Could you check a few things on this model? Use its own coordinates, in mm. A direction names the side the tool comes from. Round coordinates to 2 decimals unless told otherwise and drop trailing zeros. Write each loop counter-clockwise with the first axis right and the second up, starting at its lowest first coordinate (ties: lowest second). Pieces come first, ordered by that corner, then holes. Notation, with made-up numbers: (-7.5, 73) -> (33.5, 73) arc R24 ccw to (33.5, 85) -> close; hole circle Ø1 at (-29, 50). An arc over 180 degrees is marked (long way). Answer in a Markdown table with one row per item. Add a question column.
```python
from build123d import *

# Parameters (mm, degrees)
PAD030_DEPTH         = 10
PAD041_DEPTH         = 1
SKETCH081_R          = 4
POCKET023_DEPTH      = 16.001
POCKET023_DEPTH_BACK = 16.001


with BuildPart() as part:
    # Sketch066 → Pad030 (new body, symmetric)
    with BuildSketch(Plane.YZ):
        with BuildLine():
            ThreePointArc((54.1777871717, -5.4865141741), (68, 0), (54.1777871717, 5.4865141741))
            ThreePointArc((47.2218073921, 2.3498355523), (51.010737248, 3.2286263383), (54.1777871717, 5.4865141741))
            Line((47.2218073921, 2.3498355523), (15.1843604449, 1.3183803873))
            Line((17.6038721988, 3.8988686334), (15.1843604449, 1.3183803873))
            Line((-12.580488246, 2.9270741413), (17.6038721988, 3.8988686334))
            Line((-10, 0.5075623873), (-12.580488246, 2.9270741413))
            Line((-10, 0.5075623873), (-18, 0.25))
            ThreePointArc((-13.7330991232, 6), (-16.8683496754, 3.8684055277), (-18, 0.25))
            Line((-13.7330991232, 6), (12.3912565298, 13))
            Line((12.3912565298, 13), (103.7477270849, 13))
            ThreePointArc((107.6207104311, 8), (110.7829880912, 14.4494897428), (103.7477270849, 13))
            Line((73.7477270849, 8), (107.6207104311, 8))
            ThreePointArc((73.7477270849, 8), (72.0744070318, 7.095445115), (71.9146968069, 5.2))
            ThreePointArc((71.9146968069, -5.2), (73, 0), (71.9146968069, 5.2))
            ThreePointArc((71.9146968069, -5.2), (72.0744070318, -7.095445115), (73.7477270849, -8))
            Line((73.7477270849, -8), (107.6207104311, -8))
            ThreePointArc((103.7477270849, -13), (110.7829880912, -14.4494897428), (107.6207104311, -8))
            Line((12.3912565298, -13), (103.7477270849, -13))
            Line((-13.7330991232, -6), (12.3912565298, -13))
            ThreePointArc((-18, -0.25), (-16.8683496754, -3.8684055277), (-13.7330991232, -6))
            Line((-18, -0.25), (-10, -0.5075623873))
            Line((-10, -0.5075623873), (-12.580488246, -2.9270741413))
            Line((-12.580488246, -2.9270741413), (17.6038721988, -3.8988686334))
            Line((17.6038721988, -3.8988686334), (15.1843604449, -1.3183803873))
            Line((15.1843604449, -1.3183803873), (47.2218073921, -2.3498355523))
            ThreePointArc((54.1777871717, -5.4865141741), (51.010737248, -3.2286263383), (47.2218073921, -2.3498355523))
        make_face()
    extrude(amount=PAD030_DEPTH, both=True)

    # Sketch082 (on Face28 of Pad030) → Pad041 (join)
    with BuildSketch(Plane.YZ.offset(10)):
        Polygon((-12.580488246, 2.9270741413), (-10, 0.5075623873), (15.1843604449, 1.3183803873), (17.6038721988, 3.8988686334), align=None)
        Polygon((-10, -0.5075623873), (15.1843604449, -1.3183803873), (17.6038721988, -3.8988686334), (-12.580488246, -2.9270741413), align=None)
    extrude(amount=-PAD041_DEPTH)

    # Sketch081 → Pocket023 (cut, two sides)
    with BuildSketch(Plane.XY) as pocket023_sk:
        Circle(SKETCH081_R)
    extrude(amount=-POCKET023_DEPTH, mode=Mode.SUBTRACT)
    extrude(pocket023_sk.sketch, amount=POCKET023_DEPTH_BACK, mode=Mode.SUBTRACT)


with BuildPart() as part_1:
    # Body021 placement: moved
    add(part.part.moved(Location((0, -2, 2.5))))


solid = part_1.part
```
(1) I need wall thicknesses on L1, parallel to Z at x = 4.25, y = 58; L2, parallel to Z at x = 5.5, y = -14; L3, parallel to Z at x = -6, y = 23. Which ranges of each line are inside material? Lowest first, please.
(2) Suppose I cut it at A-A, the plane y = 58. Please give me the cut outline in (x, z), then the cut area to 3 significant figures.
(3) If we mould it in two halves opening along Z, with no side actions, what happens to faces 6 (the face through (-0.521, 1.966, 8.58)), 7 (the face through (0.14, 70.06, -4.57)), 8 (the face through (-2.082, -5.756, 11.173)), 9 (the face through (-0.367, 14.411, 5.127))? For each: pulls with the +Z half, pulls with the -Z half, needs draft (parallel to the pull), parting line crosses it, or undercut.
(4) On a 3-axis mill with a long thin cutter (end or side, diameter ignored), from which of +Z, -Z, +X, -X, +Y, -Y can I reach the whole of each face in a straight line? I mean faces 1 (the face through (-2.082, -5.756, -6.173)), 2 (the face through (10, 29, 6)), 3 (the face through (0.14, 48.961, 5.706)), 4 (the face through (0, 88, 10.5)), 5 (the face through (9, 1, 0)). Say none if no direction works.
(5) Suppose I cut it at C-C, the plane x = -0.5. State how many separate pieces and enclosed holes the cut face has, then the cut area to 3 significant figures.
(6) Suppose I cut it at B-B, the plane y = -2. Please give me the cut outline in (x, z), then the cut area to 3 significant figures.
(7) For P1, Ø1, axis at x = 3, z = 12.5, coming from the -Y side; P2, Ø8, axis at x = -6.5, y = 94, coming from the +Z side; P3, Ø12, axis at x = -6, y = 69.5, coming from the -Z side, each with a flat end and sliding along its axis, tell me the tip position at first contact or that it passes through.
Response:
| question | item | result |
|---|---|---|
| 1 | L1 | -10.5 to -5.5, 10.5 to 15.5 |
| 1 | L2 | -3.96 to -0.45, 0.12 to 2.06, 2.94 to 4.88, 5.45 to 8.96 |
| 1 | L3 | -10.5 to 0.87, 4.13 to 15.5 |
| 2 | outline | (-10, -10.5) -> (10, -10.5) -> (10, -5.5) -> (-10, -5.5) -> close; (-10, 10.5) -> (10, 10.5) -> (10, 15.5) -> (-10, 15.5) -> close |
| 2 | area | 200 mm² |
| 3 | face 6 | needs draft |
| 3 | face 7 | undercut |
| 3 | face 8 | pulls with the +Z half |
| 3 | face 9 | undercut |
| 4 | face 1 | -Z, +X, -X, -Y |
| 4 | face 2 | +Z, -Z, +X, +Y, -Y |
| 4 | face 3 | +X, -X |
| 4 | face 4 | +X, -X, +Y |
| 4 | face 5 | -X |
| 5 | separate pieces | 3 |
| 5 | enclosed holes | 0 |
| 5 | area | 1,880 mm² |
| 6 | outline | (-10, -7.18) -> (-4, -7.18) -> (-4, -0.83) -> (-10, -0.83) -> close; (-10, 5.83) -> (-4, 5.83) -> (-4, 12.18) -> (-10, 12.18) -> close; (4, -7.18) -> (10, -7.18) -> (10, 1.67) -> (9, 1.67) -> (9, -0.83) -> (4, -0.83) -> close; (4, 5.83) -> (9, 5.83) -> (9, 3.33) -> (10, 3.33) -> (10, 12.18) -> (4, 12.18) -> close |
| 6 | area | 157 mm² |
| 7 | P1 | y = -0.06 |
| 7 | P2 | z = 15.5 |
| 7 | P3 | z = -10.5 |
